```python
from build123d import *

# Parameters (mm, degrees)
SKETCH2_R               = 1.7
SKETCH2_R_2             = 4.5
BOSS_EXTRUDE1_DEPTH     = 6
FILLET1_R               = 10
CUT_EXTRUDE2_DEPTH      = 138.309868546
CUT_EXTRUDE2_DEPTH_BACK = 138.309868546
SKETCH7_R               = 2.5


with BuildPart() as part:
    # Sketch2 → Boss-Extrude1 (new body)
    with BuildSketch(Plane(origin=(0, 0, 0), x_dir=(1, 0, 0), z_dir=(0, 1, 0))):
        with BuildLine():
            Line((82.701229094, 71.670763572), (23.580603164, 14.468001358))
            Line((23.580603164, 14.468001358), (14.468001358, 23.580603164))
            Line((14.468001358, 23.580603164), (71.670763572, 82.701229094))
            ThreePointArc((71.670763572, 82.701229094), (72.579468699, 84.002771186), (73.034411761, 85.523555075))
            ThreePointArc((73.034411761, 85.523555075), (74.120868496, 87.776797037), (76.333333333, 88.944053189))
            ThreePointArc((76.333333333, 88.944053189), (77.868327334, 89.470595445), (79.153846154, 90.460996723))
            ThreePointArc((79.153846154, 90.460996723), (79.343145751, 90.656854249), (79.539003277, 90.846153846))
            ThreePointArc((79.539003277, 90.846153846), (80.529404555, 92.131672666), (81.055946811, 93.666666667))
            ThreePointArc((81.055946811, 93.666666667), (85, 97), (88.944053189, 93.666666667))
            ThreePointArc((88.944053189, 93.666666667), (89.470595445, 92.131672666), (90.460996723, 90.846153846))
            ThreePointArc((90.460996723, 90.846153846), (90.656854249, 90.656854249), (90.846153846, 90.460996723))
            ThreePointArc((90.846153846, 90.460996723), (92.131672666, 89.470595445), (93.666666667, 88.944053189))
            ThreePointArc((93.666666667, 88.944053189), (97, 85), (93.666666667, 81.055946811))
            ThreePointArc((93.666666667, 81.055946811), (92.131672666, 80.529404555), (90.846153846, 79.539003277))
            ThreePointArc((90.846153846, 79.539003277), (90.656854249, 79.343145751), (90.460996723, 79.153846154))
            ThreePointArc((90.460996723, 79.153846154), (89.470595445, 77.868327334), (88.944053189, 76.333333333))
            ThreePointArc((88.944053189, 76.333333333), (87.776797037, 74.120868496), (85.523555075, 73.034411761))
            ThreePointArc((85.523555075, 73.034411761), (84.002771186, 72.579468699), (82.701229094, 71.670763572))
        make_face()
        with Locations(Location((85, 93, 0), (0, 0, 270))):
            Circle(SKETCH2_R, mode=Mode.SUBTRACT)
        with Locations(Location((93, 85, 0), (0, 0, 270))):
            Circle(SKETCH2_R, mode=Mode.SUBTRACT)
        with Locations(Location((85, 77, 0), (0, 0, 270))):
            Circle(SKETCH2_R, mode=Mode.SUBTRACT)
        with Locations(Location((77, 85, 0), (0, 0, 270))):
            Circle(SKETCH2_R, mode=Mode.SUBTRACT)
        with Locations(Location((85, 85, 0), (0, 0, 270))):
            Circle(SKETCH2_R_2, mode=Mode.SUBTRACT)
    extrude(amount=BOSS_EXTRUDE1_DEPTH)

    # Fillet1
    # the kernel refuses this fillet: 10 mm, written as the material it takes off along each edge
    with BuildSketch(Plane(origin=(23.580603164, -24.591214075, -14.468001358), x_dir=(0.71866742198992, 0, -0.6953539649490483), z_dir=(0, 1, 0)), Plane(origin=(14.468001358, -24.591214075, -23.580603164), x_dir=(0.7071067811865477, 0, 0.7071067811865475), z_dir=(0, 1, 0))) as fillet1_piece_1:
        with BuildLine():
            CenterArc((FILLET1_R * 0.983648563013, FILLET1_R), FILLET1_R, 180.944569645, 89.055430355)
            Line((-FILLET1_R * 0.0162155484343, FILLET1_R * 0.983514896433), (0, 0))
            Line((0, 0), (FILLET1_R * 0.983648563013, 0))
        make_face()
    extrude(amount=55.182428151, mode=Mode.SUBTRACT)

    # Sketch7 → Cut-Extrude2 (cut, two sides: drawn at the far end of the back side and taken through both)
    with BuildSketch(Plane(origin=(0, 0, 0), x_dir=(1, 0, 0), z_dir=(0, 1, 0)).offset(-CUT_EXTRUDE2_DEPTH_BACK)):
        with Locations(Location((24.748737342, 24.748737342, 0), (0, 0, 270))):
            Circle(SKETCH7_R)
        with Locations(Location((31.819805153, 31.819805153, 0), (0, 0, 270))):
            Circle(SKETCH7_R)
    extrude(amount=CUT_EXTRUDE2_DEPTH + CUT_EXTRUDE2_DEPTH_BACK, mode=Mode.SUBTRACT)


solid = part.part
```
The model under review builds one solid part; all positions refer to its coordinate system, in mm. Round coordinates to 2 decimals unless told otherwise and drop trailing zeros. Order: outer loops, then holes, each group sorted by start corner. A loop starts at its lowest first (then second) coordinate and runs counter-clockwise, first axis right, second up. Notation, with made-up numbers: (80, 19) -> (91, 19) arc R25 cw to (91, 44) -> close; hole circle Ø4 at (61.25, 80.25). An arc over 180 degrees is marked (long way). Use a Markdown table: item, result.
Q1. We need section B-B on z = -45.5. Write out the cut boundary in (x, y), then the cut area to 3 significant figures.
Values:
| item | result |
|---|---|
| outline | (35.68, 0) -> (55.65, 0) -> (55.65, 6) -> (35.68, 6) -> close |
| area | 120 mm^2 |
Q2. We need section A-A on y = 1.2. Write out the cut boundary in (x, z), then the cut area to 3 significant figures.
Values:
| item | result |
|---|---|
| outline | (19.44, -19.44) arc R10 ccw to (21.31, -30.65) -> (71.67, -82.7) arc R5 cw to (73.03, -85.52) arc R4 ccw to (76.33, -88.94) arc R5 cw to (79.15, -90.46) arc R8 ccw to (79.54, -90.85) arc R5 cw to (81.06, -93.67) arc R4 ccw to (88.94, -93.67) arc R5 cw to (90.46, -90.85) arc R8 ccw to (90.85, -90.46) arc R5 cw to (93.67, -88.94) arc R4 ccw to (93.67, -81.06) arc R5 cw to (90.85, -79.54) arc R8 ccw to (90.46, -79.15) arc R5 cw to (88.94, -76.33) arc R4 ccw to (85.52, -73.03) arc R5 cw to (82.7, -71.67) -> (30.65, -21.31) arc R10 ccw to start; hole circle Ø5 at (24.75, -24.75); hole circle Ø5 at (31.82, -31.82); hole circle Ø3.4 at (77, -85); hole circle Ø9 at (85, -85); hole circle Ø3.4 at (85, -93); hole circle Ø3.4 at (85, -77); hole circle Ø3.4 at (93, -85) |
| area | 1,340 mm^2 |
Q3. Clearance check with flat-ended pins moving along their axes: P1, Ø1, axis at y = 2.5, z = -37.5, coming from the +X side; P2, Ø1.5, axis at x = 31, y = 3.5, coming from the +Z side; P3, Ø2.5, axis at x = 93, z = -85, coming from the -Y side; P4, Ø1.5, axis at x = 70.5, y = 4, coming from the -Z side. State where each tip first meets the part, or that it passes through.
Values:
| item | result |
|---|---|
| P1 | stops at x = 47.9 |
| P2 | stops at z = -20.94 |
| P3 | passes through |
| P4 | stops at z = -82.27 |
Q4. For line 1 (Z direction, x = 84.5, y = 4.3); line 2 (Z direction, x = 86.5, y = 3.2); line 3 (X direction, y = 2.1, z = -77), list the stretches that pass through material, from the lowest coordinate up.
Values:
| item | result |
|---|---|
| line 1 | z = -96.97 to -94.62, -91.38 to -89.47, -80.53 to -78.62, -75.38 to -72.79 |
| line 2 | z = -96.71 to -93.8, -92.2 to -89.24, -80.76 to -77.8, -76.2 to -73.29 |
| line 3 | x = 66.15 to 83.3, 86.7 to 89.1 |
Q5. We need section C-C on z = -36.5. Write out the cut boundary in (x, y), then the cut area to 3 significant figures.
Values:
| item | result |
|---|---|
| outline | (26.97, 0) -> (46.35, 0) -> (46.35, 6) -> (26.97, 6) -> close |
| area | 116 mm^2 |
Q6. Mouldability with a two-part tool opening along Z and no side actions: class faces 1 (the cylindrical face through (87.802, 2.958, -74.146)), 2 (the cylindrical face through (30.86, 2.96, -29.51)), 3 (the flat face through (46.137, 2.958, -56.311)) as +Z half, -Z half, draft (parallel to the pull), parting line (faces both ways), or undercut.
Values:
| item | result |
|---|---|
| face 1 | +Z half |
| face 2 | undercut |
| face 3 | -Z half |
